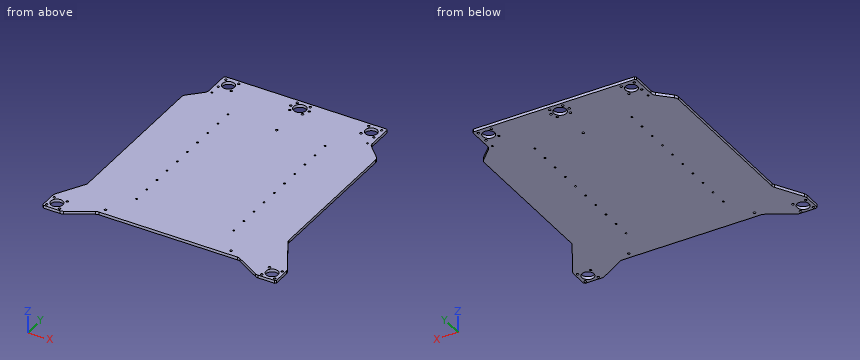
```python
from build123d import *

# Parameters (mm, degrees)
SKETCH1_W           = 170
SKETCH1_H           = 340
BOSS_EXTRUDE1_DEPTH = 5
SKETCH2_R           = 2
CUT_EXTRUDE1_DEPTH  = 241.468293128
SKETCH3_R           = 2
SKETCH3_R_2         = 10.55
SKETCH3_R_3         = 1.5
BOSS_EXTRUDE2_DEPTH = 5
CHAMFER3_SIZE       = 5
FILLET1_R           = 10
CHAMFER2_SIZE       = 2
MIRROR2_OUTLINE_R   = 2
MIRROR2_OUTLINE_R_2 = 1.5
MIRROR2_OUTLINE_R_3 = 10.55
MIRROR2_DEPTH       = 5
SKETCH5_R           = 10.55
SKETCH5_R_2         = 2
BOSS_EXTRUDE3_DEPTH = 5
CHAMFER4_SIZE       = 2
FILLET2_R           = 10
SKETCH4_R           = 1.5
CUT_EXTRUDE2_DEPTH  = 325.156212342


# Read off the part's stored shape, not the designer's step: Mirror2
with BuildPart() as part:
    # Sketch1 → Boss-Extrude1 (new body)
    with BuildSketch(Plane.XY):
        with Locations((-85, 0)):
            Rectangle(SKETCH1_W, SKETCH1_H)
    extrude(amount=BOSS_EXTRUDE1_DEPTH)

    # Sketch2 → Cut-Extrude1 (cut, through all)
    with BuildSketch(Plane.XY.offset(5)):
        with Locations((-110, -160)):
            Circle(SKETCH2_R)
        with Locations((0, 160)):
            Circle(SKETCH2_R)
    extrude(amount=-CUT_EXTRUDE1_DEPTH, mode=Mode.SUBTRACT)

    # Sketch3 → Boss-Extrude2 (add)
    with BuildSketch(Plane.XY.offset(5)):
        with BuildLine():
            Line((-170, 170), (-143, 196.8))
            Line((-143, 196.8), (-143, 246.8))
            Line((-143, 246.8), (0, 246.8))
            Line((0, 246.8), (0, 239.85))
            ThreePointArc((0, 239.85), (-11.05, 228.8), (0, 217.75))
            Line((0, 217.75), (0, 170))
            Line((0, 170), (-170, 170))
        make_face()
        with Locations((-11.313708499, 240.113708499)):
            Circle(SKETCH3_R, mode=Mode.SUBTRACT)
        with Locations((-11.313708499, 217.486291501)):
            Circle(SKETCH3_R, mode=Mode.SUBTRACT)
        with Locations((-16, 228.8)):
            Circle(SKETCH3_R, mode=Mode.SUBTRACT)
        with Locations((-125, 228.8)):
            Circle(SKETCH3_R_2, mode=Mode.SUBTRACT)
        with Locations((-136.313708499, 240.113708499)):
            Circle(SKETCH3_R, mode=Mode.SUBTRACT)
        with Locations((-113.686291501, 240.113708499)):
            Circle(SKETCH3_R, mode=Mode.SUBTRACT)
        with Locations((-136.313708499, 217.486291501)):
            Circle(SKETCH3_R, mode=Mode.SUBTRACT)
        with Locations((-113.686291501, 217.486291501)):
            Circle(SKETCH3_R, mode=Mode.SUBTRACT)
        with Locations((-136.313708499, 198.8)):
            Circle(SKETCH3_R_3, mode=Mode.SUBTRACT)
    extrude(amount=-BOSS_EXTRUDE2_DEPTH)

    # Chamfer3
    chamfer3_edges = [part.edges().sort_by_distance(p)[0] for p in [
        (-170, -170, 2.5),
    ]]
    chamfer(chamfer3_edges, length=CHAMFER3_SIZE)

    # Fillet1
    fillet1_edges = [part.edges().sort_by_distance(p)[0] for p in [
        (-143, 196.8, 2.5),
        (-170, 170, 2.5),
    ]]
    fillet(fillet1_edges, radius=FILLET1_R)

    # Chamfer2
    chamfer2_edges = [part.edges().sort_by_distance(p)[0] for p in [
        (-143, 246.8, 2.5),
    ]]
    chamfer(chamfer2_edges, length=CHAMFER2_SIZE)

    # Mirror2 outline → Mirror2 (add)
    with BuildSketch(Plane.XY):
        with BuildLine():
            Line((0, -170), (165, -170))
            Line((165, -170), (170, -165))
            Line((170, -165), (170, 165.836071225))
            ThreePointArc((170, 165.836071225), (169.231666328, 169.680071331), (167.044732637, 172.933376494))
            Line((167.044732637, 172.933376494), (145.955267363, 193.866623506))
            ThreePointArc((145.955267363, 193.866623506), (143.768333672, 197.119928669), (143, 200.963928775))
            Line((143, 200.963928775), (143, 244.8))
            Line((143, 244.8), (141, 246.8))
            Line((141, 246.8), (0, 246.8))
            Line((0, 246.8), (0, 239.85))
            ThreePointArc((0, 239.85), (11.05, 228.8), (0, 217.75))
            Line((0, 217.75), (0, 162))
            ThreePointArc((0, 162), (2, 160), (0, 158))
            Line((0, 158), (0, -170))
        make_face()
        with Locations((110, -160)):
            Circle(MIRROR2_OUTLINE_R, mode=Mode.SUBTRACT)
        with Locations((11.313708499, 217.486291501)):
            Circle(MIRROR2_OUTLINE_R, mode=Mode.SUBTRACT)
        with Locations((11.313708499, 240.113708499)):
            Circle(MIRROR2_OUTLINE_R, mode=Mode.SUBTRACT)
        with Locations((16, 228.8)):
            Circle(MIRROR2_OUTLINE_R, mode=Mode.SUBTRACT)
        with Locations((113.686291501, 217.486291501)):
            Circle(MIRROR2_OUTLINE_R, mode=Mode.SUBTRACT)
        with Locations((113.686291501, 240.113708499)):
            Circle(MIRROR2_OUTLINE_R, mode=Mode.SUBTRACT)
        with Locations((136.313708499, 198.8)):
            Circle(MIRROR2_OUTLINE_R_2, mode=Mode.SUBTRACT)
        with Locations((136.313708499, 217.486291501)):
            Circle(MIRROR2_OUTLINE_R, mode=Mode.SUBTRACT)
        with Locations((125, 228.8)):
            Circle(MIRROR2_OUTLINE_R_3, mode=Mode.SUBTRACT)
        with Locations((136.313708499, 240.113708499)):
            Circle(MIRROR2_OUTLINE_R, mode=Mode.SUBTRACT)
    extrude(amount=MIRROR2_DEPTH)

    # Sketch5 → Boss-Extrude3 (add)
    # profile 1 of 2: a face of its own
    with BuildSketch(Plane.XY.offset(5)):
        Polygon((-198.8, -162.75), (-198.8, -196.75), (-164.8, -196.75), (-118.467640898, -170), (-170, -112.866936742), align=None)
        with Locations((-182.8, -180.75)):
            Circle(SKETCH5_R, mode=Mode.SUBTRACT)
        with Locations((-194.113708499, -169.436291501)):
            Circle(SKETCH5_R_2, mode=Mode.SUBTRACT)
        with Locations((-171.486291501, -169.436291501)):
            Circle(SKETCH5_R_2, mode=Mode.SUBTRACT)
        with Locations((-171.486291501, -192.063708499)):
            Circle(SKETCH5_R_2, mode=Mode.SUBTRACT)
        with Locations((-194.113708499, -192.063708499)):
            Circle(SKETCH5_R_2, mode=Mode.SUBTRACT)
    # profile 2 of 2: a face of its own
    with BuildSketch(Plane.XY.offset(5)):
        Polygon((176.1, -196.75), (210.1, -196.75), (210.1, -162.75), (170, -93.294762616), (129.767640898, -170), align=None)
        with Locations((194.1, -180.75)):
            Circle(SKETCH5_R, mode=Mode.SUBTRACT)
        with Locations((205.413708499, -192.063708499)):
            Circle(SKETCH5_R_2, mode=Mode.SUBTRACT)
        with Locations((205.413708499, -169.436291501)):
            Circle(SKETCH5_R_2, mode=Mode.SUBTRACT)
        with Locations((182.786291501, -169.436291501)):
            Circle(SKETCH5_R_2, mode=Mode.SUBTRACT)
        with Locations((182.786291501, -192.063708499)):
            Circle(SKETCH5_R_2, mode=Mode.SUBTRACT)
    extrude(amount=-BOSS_EXTRUDE3_DEPTH)

    # Chamfer4
    chamfer4_edges = [part.edges().sort_by_distance(p)[0] for p in [
        (-198.8, -196.75, 2.5),
        (210.1, -196.75, 2.5),
    ]]
    chamfer(chamfer4_edges, length=CHAMFER4_SIZE)

    # Fillet2
    fillet2_edges = [part.edges().sort_by_distance(p)[0] for p in [
        (-198.8, -162.75, 2.5),
        (-170, -112.866936742, 2.5),
        (-118.467640898, -170, 2.5),
        (-164.8, -196.75, 2.5),
        (176.1, -196.75, 2.5),
        (129.767640898, -170, 2.5),
        (170, -93.294762616, 2.5),
        (210.1, -162.75, 2.5),
    ]]
    fillet(fillet2_edges, radius=FILLET2_R)

    # Sketch4 → Cut-Extrude2 (cut, through all)
    with BuildSketch(Plane.XY.offset(5)):
        with Locations((-85, 160)):
            Circle(SKETCH4_R)
        with Locations((-85, 130)):
            Circle(SKETCH4_R)
        with Locations((-85, 100)):
            Circle(SKETCH4_R)
        with Locations((-85, 70)):
            Circle(SKETCH4_R)
        with Locations((-85, 40)):
            Circle(SKETCH4_R)
        with Locations((-85, 10)):
            Circle(SKETCH4_R)
        with Locations((-85, -20)):
            Circle(SKETCH4_R)
        with Locations((-85, -50)):
            Circle(SKETCH4_R)
        with Locations((-85, -80)):
            Circle(SKETCH4_R)
        with Locations((-85, -110)):
            Circle(SKETCH4_R)
    cut_extrude2 = extrude(amount=-CUT_EXTRUDE2_DEPTH, mode=Mode.SUBTRACT)

    # Mirror3: Cut-Extrude2 across plane
    add(cut_extrude2.mirror(Plane(origin=(0, 0, 0), x_dir=(0, 0, 1), z_dir=(1, 0, 0))), mode=Mode.SUBTRACT)


solid = part.part
```
Read the model definition and answer for the solid it produces. Units are mm, in the model's axes. Coordinates: 2 decimals unless noted, no trailing zeros. Write each loop counter-clockwise with the first axis right and the second up, starting at its lowest first coordinate (ties: lowest second). Pieces come first, ordered by that corner, then holes. Notation, with made-up numbers: (22.5, 72) -> (31.5, 72) arc R18 cw to (31.5, 77) -> close; hole circle Ø9 at (68, 49.25). An arc over 180 degrees is marked (long way). Answer as a JSON object with one key per item and string values.
Q1. The part is cut by section C-C on y = 151.5. Give the vertices of the cut face in (x, z).
The answers:
{"outline": "(-170, 0) -> (170, 0) -> (170, 5) -> (-170, 5) -> close"}
Q2. The part is cut by section A-A on y = -180.75. Give the vertices of the cut face in (x, z).
The answers:
{"outline": "(-198.8, 0) -> (-193.35, 0) -> (-193.35, 5) -> (-198.8, 5) -> close; (-172.25, 0) -> (-137.09, 0) -> (-137.09, 5) -> (-172.25, 5) -> close; (148.39, 0) -> (183.55, 0) -> (183.55, 5) -> (148.39, 5) -> close; (204.65, 0) -> (210.1, 0) -> (210.1, 5) -> (204.65, 5) -> close"}
Q3. Consider line 1 (X direction, y = 70, z = 1.3); line 2 (Y direction, x = 0, z = 1); line 3 (Y direction, x = 183, z = 3.75). Determine where each line is inside the solid, lowest interval first. Write a range as [from, to].
The answers:
{"line 1": "x = [-170, -86.5], [-83.5, 83.5], [86.5, 170]", "line 2": "y = [-170, 158], [162, 217.75], [239.85, 246.8]", "line 3": "y = [-196.75, -194.05], [-190.08, -171.42], [-167.45, -115.81]"}
Q4. Flat-ended cylindrical pins translate along their axes: pin 1 Ø4 at (x, y) = (85, -50) entering from +Z; pin 2 Ø2.5 at (x, y) = (-85, 130) entering from -Z; pin 3 Ø2 at (x, z) = (21.5, 4) entering from -Y. Find the tip coordinate at first contact, or state that the pin passes through.
The answers:
{"pin 1": "stops at z = 5", "pin 2": "passes through", "pin 3": "stops at y = -170"}
Q5. The part is cut by section B-B on x = 194.1. Give the vertices of the cut face in (y, z), then the cut area to 3 significant figures.
The answers:
{"outline": "(-196.75, 0) -> (-191.3, 0) -> (-191.3, 5) -> (-196.75, 5) -> close; (-170.2, 0) -> (-135.04, 0) -> (-135.04, 5) -> (-170.2, 5) -> close", "area": "203 mm2"}
Q6. The part is cut by section D-D on x = 38.5. Give the vertices of the cut face in (y, z).
The answers:
{"outline": "(-170, 0) -> (246.8, 0) -> (246.8, 5) -> (-170, 5) -> close"}
